Could you check a few things on this model? Use its own coordinates, in mm. Coordinates: 2 decimals unless noted, no trailing zeros. Order: outer loops, then holes, each group sorted by start corner. A loop starts at its lowest first (then second) coordinate and runs counter-clockwise, first axis right, second up. Notation, with made-up numbers: (0, -7.75) - (58, -7.75) arc R23 ccw to (58, 31.25) - close; hole circle Ø7 at (0.5, -5.5). An arc over 180 degrees is marked (long way). Answer as a JSON object with one key per item and string values. Group by question number.
(1) Imagine slicing it at D-D, the plane x = 87. Write out the boundary of the cut face in (y, z) (3 decimals), and give its area (3 significant figures).
(2) Imagine slicing it at B-B, the plane z = 1.4. Write out the boundary of the cut face in (x, y) (3 decimals), and give its area (3 significant figures).
(3) Please list where these lines run through material, in increasing order: probe 1 along Y at (x, z) = (26, 1.3); probe 2 along X at (y, z) = (17, 1); probe 3 along X at (y, z) = (15, 0.2).
(4) Imagine slicing it at A-A, the plane y = 14.5. Write out the boundary of the cut face in (x, z) (3 decimals), and give its area (3 significant figures).
(5) Will these pins go through, and if not, where does the flat tip stop? P1, Ø4.5, axis at x = 27.9, y = 15.88, coming from the +Z side; P2, Ø1, axis at x = 84.5, z = 2.5, coming from the +Y side.
(6) Imagine slicing it at C-C, the plane y = 36. Write out the boundary of the cut face in (x, z) (3 decimals).
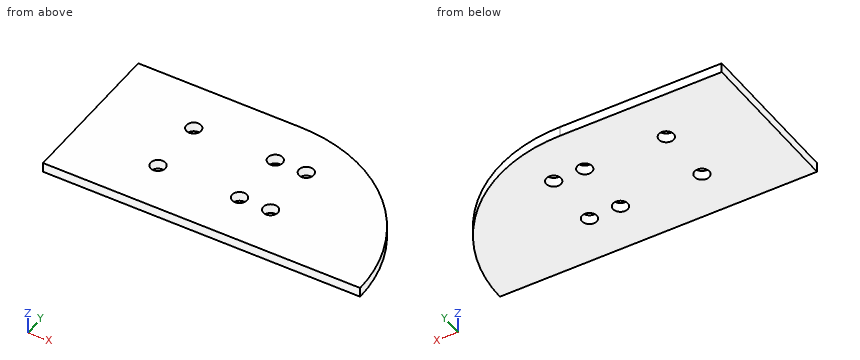
from build123d import *

# Parameters (mm, degrees)
BOSS_EXTRUDE1_DEPTH     = 3.175
SKETCH3_R               = 2.413
CUT_EXTRUDE1_DEPTH      = 1
CUT_EXTRUDE1_DEPTH_BACK = 4.175


with BuildPart() as part:
    # Sketch1 → Boss-Extrude1 (new body)
    with BuildSketch(Plane.XY):
        with BuildLine():
            Line((0, 50.8), (0, 0))
            Line((0, 0), (103.778975516, 0))
            ThreePointArc((103.778975516, 0), (88.9, 35.921024484), (52.978975516, 50.8))
            Line((52.978975516, 50.8), (0, 50.8))
        make_face()
    extrude(amount=BOSS_EXTRUDE1_DEPTH)

    # Sketch3 → Cut-Extrude1 (cut, two sides)
    with BuildSketch(Plane.XY.offset(3.175)) as cut_extrude1_sk:
        with Locations((64.726475516, 15.875)):
            Circle(SKETCH3_R)
        with Locations((64.726475516, 34.925)):
            Circle(SKETCH3_R)
        with Locations((27.896475516, 15.875)):
            Circle(SKETCH3_R)
        with Locations((27.896475516, 34.925)):
            Circle(SKETCH3_R)
        with Locations((54.566475516, 34.925)):
            Circle(SKETCH3_R)
        with Locations((54.566475516, 15.875)):
            Circle(SKETCH3_R)
    extrude(amount=CUT_EXTRUDE1_DEPTH, mode=Mode.SUBTRACT)
    extrude(cut_extrude1_sk.sketch, amount=-CUT_EXTRUDE1_DEPTH_BACK, mode=Mode.SUBTRACT)


solid = part.part
Result set:
{
 "1": {"outline": "(0, 0) - (37.725, 0) - (37.725, 3.175) - (0, 3.175) - close", "area": "120 mm^2"},
 "2": {"outline": "(0, 0) - (103.779, 0) arc R50.8 ccw to (52.979, 50.8) - (0, 50.8) - close; hole circle Ø4.826 at (27.896, 15.875); hole circle Ø4.826 at (27.896, 34.925); hole circle Ø4.826 at (54.566, 15.875); hole circle Ø4.826 at (54.566, 34.925); hole circle Ø4.826 at (64.726, 15.875); hole circle Ø4.826 at (64.726, 34.925)", "area": "4,610 mm^2"},
 "3": {"probe 1": "y = 0 to 14.38, 17.37 to 33.43, 36.42 to 50.8", "probe 2": "x = 0 to 25.76, 30.03 to 52.43, 56.7 to 62.59, 66.86 to 100.85", "probe 3": "x = 0 to 25.65, 30.15 to 52.32, 56.82 to 62.48, 66.98 to 101.51"},
 "4": {"outline": "(0, 0) - (25.914, 0) - (25.914, 3.175) - (0, 3.175) - close; (29.879, 0) - (52.584, 0) - (52.584, 3.175) - (29.879, 3.175) - close; (56.549, 0) - (62.744, 0) - (62.744, 3.175) - (56.549, 3.175) - close; (66.709, 0) - (101.666, 0) - (101.666, 3.175) - (66.709, 3.175) - close", "area": "285 mm^2"},
 "5": {"P1": "passes through", "P2": "stops at y = 40.23"},
 "6": {"outline": "(0, 0) - (25.736, 0) - (25.736, 3.175) - (0, 3.175) - close; (30.057, 0) - (52.406, 0) - (52.406, 3.175) - (30.057, 3.175) - close; (56.727, 0) - (62.566, 0) - (62.566, 3.175) - (56.727, 3.175) - close; (66.887, 0) - (88.821, 0) - (88.821, 3.175) - (66.887, 3.175) - close"}
}
